Verification items for the finished model (mm, model axes). Face numbers are marked on the shaded views. A direction names the side the tool comes from. Round coordinates to 2 decimals unless told otherwise and drop trailing zeros. Write each loop counter-clockwise with the first axis right and the second up, starting at its lowest first coordinate (ties: lowest second). Pieces come first, ordered by that corner, then holes.
from build123d import *

# Parameters (mm, degrees)
F1_DEPTH  = 44.704
F4_D      = 6.35
F4_DEPTH  = 50.8
F6_DEPTH  = 25.4
F8_DEPTH  = 25.4
F10_DEPTH = 25.4


with BuildPart() as f1:
    # F0 (on Right) → F1 (new body)
    with BuildSketch(Plane.YZ):
        Polygon((-33.479363, 12.7), (-33.479363, 0), (61.770637, 0), (61.770637, 25.4), (10.970637, 25.4), (10.970637, 12.7), align=None)
    extrude(amount=F1_DEPTH)

    # F4
    with Locations(Plane.XY.offset(12.7)):
        with Locations((22.09222, -20.542669)):
            Hole(F4_D / 2, depth=F4_DEPTH)

    # F5 (on face) → F6 (cut)
    with BuildSketch(Plane.XY.offset(12.7)):
        Polygon((25.304057, -21.059527), (19.101784, -21.059527), (19.101784, -33.980933), (25.304057, -33.759527), align=None)
    extrude(amount=-F6_DEPTH, mode=Mode.SUBTRACT)

    # F7 (on face) → F8 (cut)
    with BuildSketch(Plane.XY.offset(25.4)):
        with BuildLine():
            ThreePointArc((0, 41.87514), (22.352, 61.643697), (44.704, 41.87514))
            Line((44.704, 41.87514), (44.704, 61.770637))
            Line((44.704, 61.770637), (0, 61.770637))
            Line((0, 61.770637), (0, 41.87514))
        make_face()
    extrude(amount=-F8_DEPTH, mode=Mode.SUBTRACT)

    # F9 (on face) → F10 (cut)
    with BuildSketch(Plane.XY.offset(25.4)):
        with BuildLine():
            ThreePointArc((30.353, 36.370637), (16.694439, 42.028199), (22.352, 28.369637))
            ThreePointArc((22.352, 28.369637), (28.009561, 30.713076), (30.353, 36.370637))
        make_face()
    extrude(amount=-F10_DEPTH, mode=Mode.SUBTRACT)


solid = f1.part
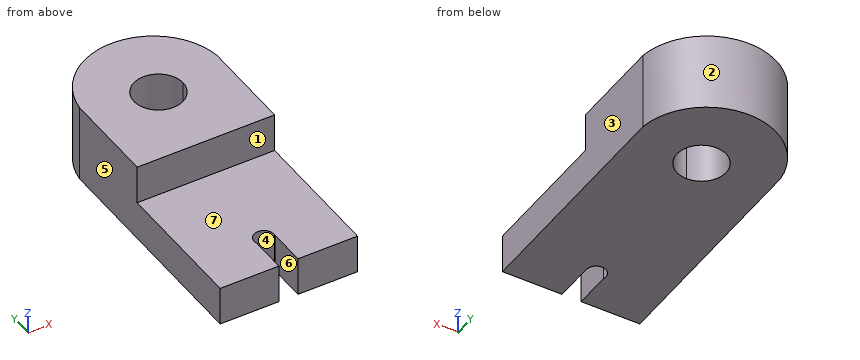
Q1. Sectioned sample at B-B (y = -23.5). Enter the section's corners in (x, z), plus the area to 3 significant figures.
Recorded:
outline: (0, 0) - (19.1, 0) - (19.1, 12.7) - (0, 12.7) - close; (25.3, 0) - (44.7, 0) - (44.7, 12.7) - (25.3, 12.7) - close
area: 489 mm2
Q2. Depth check by flat-ended pin: P1, Ø10, axis at x = 33, z = 19.5, coming from the -Y side. Enter the tip coordinate at first touch or a pass-through.
Recorded:
P1: stops at y = 10.97
Q3. Material ranges on line 1 along Z through (x, y) = (10, -11); line 2 along Y through (x, z) = (15, 18.25); line 3 along X through (y, z) = (41.5, 1.5), recorded low to high.
Recorded:
line 1: z = 0 to 12.7
line 2: y = 10.97 to 33.21, 39.53 to 60.41
line 3: x = 0 to 16.21, 28.49 to 44.7
Q4. Tool access check on the marked faces 5, 6 and 7. Record the directions out of +Z, -Z, +X, -X, +Y, -Y that give a thin tool (end or side, any length) a straight path to the whole face; none if there is none.
Recorded:
face 5: +Z, -Z, -X, +Y, -Y
face 6: +Z, -Z, -Y
face 7: +Z, +X, -X, -Y
Q5. Release check for a two-part mould opening along Y. For the marked faces 1, 2, 3 and 4 record: released by +Y, released by -Y, zero draft, split by the parting line, or undercut.
Recorded:
face 1: released by -Y
face 2: released by +Y
face 3: zero draft
face 4: undercut
Q6. Sectioned sample at C-C (x = 21). Enter the section's corners in (y, z).
Recorded:
outline: (-17.56, 0) - (28.48, 0) - (28.48, 25.4) - (10.97, 25.4) - (10.97, 12.7) - (-17.56, 12.7) - close; (44.26, 0) - (61.6, 0) - (61.6, 25.4) - (44.26, 25.4) - close
Q7. Sectioned sample at D-D (y = 4). Enter the section's corners in (x, z).
Recorded:
outline: (0, 0) - (44.7, 0) - (44.7, 12.7) - (0, 12.7) - close
Q8. Sectioned sample at A-A (z = 4.75). Enter the section's corners in (x, y) (3 decimals).
Recorded:
outline: (0, -33.479) - (19.102, -33.479) - (19.102, -21.609) arc R3.175 cw (long way) to (25.225, -21.06) - (25.304, -21.06) - (25.304, -33.479) - (44.704, -33.479) - (44.704, 41.875) arc R22.521 ccw to (0, 41.875) - close; hole (22.352, 28.37) arc R8.001 ccw to (30.353, 36.371) arc R8.001 ccw (long way) to start
